Design review of the part built by this model. Coordinates are the model's own, in mm. Face numbers are marked on the shaded views. A direction names the side the tool comes from. Coordinates: 2 decimals unless noted, no trailing zeros. Order: outer loops, then holes, each group sorted by start corner. A loop starts at its lowest first (then second) coordinate and runs counter-clockwise, first axis right, second up. Notation, with made-up numbers: (23, 74.5) -> (68, 74.5) arc R17 ccw to (68, 83.5) -> close; hole circle Ø8 at (48.25, 78.25). An arc over 180 degrees is marked (long way). Use a Markdown table: item, result. Add a question column.
Q1. Machinability: for the marked faces 4 and 5, which of the approach directions +Z, -Z, +X, -X, +Y, -Y give a long, thin tool a straight path to every point of the face, cutting with its end or side? Answer none if there is none.
Q2. The part is to be moulded in two halves that separate along Y. For the marked faces 1, 2 and 3, say which applies: pulls with the +Y half, pulls with the -Y half, needs draft (parallel to the pull), parting line crosses it, or undercut.
Q3. Add section C-C (y = 2). State the section outline as (x, z) points, then the cut area to 3 significant figures.
Q4. Add section A-A (x = 0). State the section outline as (y, z) points.
Q5. Insertion check: pin 1 (1 mm diameter, centred on x = 2, z = -2.5, fed in from +Y); pin 2 (9 mm diameter, centred on x = 0, y = 0, fed in from +Z); pin 3 (1.5 mm diameter, centred on y = 6, z = -1.5, fed in from -X). Each pin has a flat end and moves straight along its axis. Give the tip position at first contact, or say it passes through.
Q6. Wall thickness on probe 1 along Y at (x, z) = (0, -0.55); probe 2 along Y at (x, z) = (0, -1.8); probe 3 along Y at (x, z) = (-0.25, -0.15): over which ranges is each line inside the solid? List them lowest first.
Q7. Add section B-B (z = -2.7). State the section outline as (x, y) points, then the cut area to 3 significant figures.
Q8. Add section D-D (x = 3.25). State the section outline as (y, z) points, then the cut area to 3 significant figures.
from build123d import *

# Parameters (mm, degrees)
F0_R         = 2.75
F1_DEPTH     = 3
F2_DEPTH     = 1.5
F3_T4_DEPTH  = 26.4678686971
F3_S5_R      = 9
F3_T6_DEPTH  = 15
F3_T10_DEPTH = 20.3478228694
F3_S11_R     = 9
F3_T12_DEPTH = 12
F3_T16_DEPTH = 26.4678686971
F3_S17_R     = 9
F3_T18_DEPTH = 15
F3_T22_DEPTH = 20.3478228694
F3_S23_R     = 9
F3_T24_DEPTH = 12


# Not quite as in the source:
# - a fillet or chamfer that OpenCascade refuses, or shapes differently, is made with other operations: its cross-section is extruded or revolved along the edge and cut away or added


with BuildPart() as f1:
    # F0 (on Top) → F1 (new body)
    with BuildSketch(Plane.XY):
        with BuildLine():
            Line((-5.3326822519, 7.25), (5.3326822519, 7.25))
            ThreePointArc((5.3326822519, 7.25), (0, 9), (-5.3326822519, 7.25))
        make_face()
        with BuildLine():
            Line((-8.3927051658, 3.25), (8.3927051658, 3.25))
            ThreePointArc((8.3927051658, 3.25), (7.1481861295, 5.4684033372), (5.3326822519, 7.25))
            Line((5.3326822519, 7.25), (-5.3326822519, 7.25))
            ThreePointArc((-5.3326822519, 7.25), (-7.1481861295, 5.4684033372), (-8.3927051658, 3.25))
        make_face()
        with BuildLine():
            ThreePointArc((5.3326822519, -7.25), (7.1481861295, -5.4684033372), (8.3927051658, -3.25))
            Line((8.3927051658, -3.25), (-8.3927051658, -3.25))
            ThreePointArc((-8.3927051658, -3.25), (-7.1481861295, -5.4684033372), (-5.3326822519, -7.25))
            Line((-5.3326822519, -7.25), (5.3326822519, -7.25))
        make_face()
        with BuildLine():
            ThreePointArc((-5.3326822519, -7.25), (0, -9), (5.3326822519, -7.25))
            Line((5.3326822519, -7.25), (-5.3326822519, -7.25))
        make_face()
        with BuildLine():
            ThreePointArc((8.3927051658, -3.25), (8.8468736425, -1.6531263575), (9, 0))
            ThreePointArc((9, 0), (8.8468736425, 1.6531263575), (8.3927051658, 3.25))
            Line((8.3927051658, 3.25), (-8.3927051658, 3.25))
            ThreePointArc((-8.3927051658, 3.25), (-9, 0), (-8.3927051658, -3.25))
            Line((-8.3927051658, -3.25), (8.3927051658, -3.25))
        make_face()
        Circle(F0_R, mode=Mode.SUBTRACT)
    extrude(amount=-F1_DEPTH)

    # F0 (on Top) → F2 (cut)
    with BuildSketch(Plane.XY):
        with BuildLine():
            Line((-8.3927051658, 3.25), (8.3927051658, 3.25))
            ThreePointArc((8.3927051658, 3.25), (7.1481861295, 5.4684033372), (5.3326822519, 7.25))
            Line((5.3326822519, 7.25), (-5.3326822519, 7.25))
            ThreePointArc((-5.3326822519, 7.25), (-7.1481861295, 5.4684033372), (-8.3927051658, 3.25))
        make_face()
        with BuildLine():
            ThreePointArc((5.3326822519, -7.25), (7.1481861295, -5.4684033372), (8.3927051658, -3.25))
            Line((8.3927051658, -3.25), (-8.3927051658, -3.25))
            ThreePointArc((-8.3927051658, -3.25), (-7.1481861295, -5.4684033372), (-5.3326822519, -7.25))
            Line((-5.3326822519, -7.25), (5.3326822519, -7.25))
        make_face()
    extrude(amount=-F2_DEPTH, mode=Mode.SUBTRACT)

    # F3: fillet of radius 2 on 4 edges, made by hand


with BuildPart() as f3_tool2:
    # F3_s3 → F3_t4 (new body)
    with BuildSketch(Plane.YZ.offset(-13.2339343486)):
        with BuildLine():
            ThreePointArc((3.25, 0), (3.9617468017, -1.0811388301), (5.1864916731, -1.5))
            Line((5.1864916731, -1.5), (3.25, -1.5))
            Line((3.25, -1.5), (3.25, 0))
        make_face()
    extrude(amount=F3_T4_DEPTH)

    # F3_s5 → F3_t6 (intersect, symmetric)
    with BuildSketch(Plane.XY.offset(-0.8)):
        Circle(F3_S5_R)
    extrude(amount=F3_T6_DEPTH, both=True, mode=Mode.INTERSECT)


with BuildPart() as f1_1:
    add(f1.part)

    # F3_t1: union F3_tool2
    add(f3_tool2.part)


with BuildPart() as f3_tool8:
    # F3_s9 → F3_t10 (new body)
    with BuildSketch(Plane.YZ.offset(10.1739114347)):
        with BuildLine():
            ThreePointArc((5.3135083269, -1.5), (6.5382531983, -1.0811388301), (7.25, 0))
            Line((7.25, 0), (7.25, -1.5))
            Line((7.25, -1.5), (5.3135083269, -1.5))
        make_face()
    extrude(amount=-F3_T10_DEPTH)

    # F3_s11 → F3_t12 (intersect, symmetric)
    with BuildSketch(Plane.XY.offset(-0.8)):
        Circle(F3_S11_R)
    extrude(amount=F3_T12_DEPTH, both=True, mode=Mode.INTERSECT)


with BuildPart() as f1_2:
    add(f1_1.part)

    # F3_t7: union F3_tool8
    add(f3_tool8.part)


with BuildPart() as f3_tool14:
    # F3_s15 → F3_t16 (new body)
    with BuildSketch(Plane.YZ.offset(13.2339343486)):
        with BuildLine():
            ThreePointArc((-3.25, 0), (-3.9617468017, -1.0811388301), (-5.1864916731, -1.5))
            Line((-5.1864916731, -1.5), (-3.25, -1.5))
            Line((-3.25, -1.5), (-3.25, 0))
        make_face()
    extrude(amount=-F3_T16_DEPTH)

    # F3_s17 → F3_t18 (intersect, symmetric)
    with BuildSketch(Plane.XY.offset(-0.8)):
        Circle(F3_S17_R)
    extrude(amount=F3_T18_DEPTH, both=True, mode=Mode.INTERSECT)


with BuildPart() as f1_3:
    add(f1_2.part)

    # F3_t13: union F3_tool14
    add(f3_tool14.part)


with BuildPart() as f3_tool20:
    # F3_s21 → F3_t22 (new body)
    with BuildSketch(Plane.YZ.offset(-10.1739114347)):
        with BuildLine():
            ThreePointArc((-5.3135083269, -1.5), (-6.5382531983, -1.0811388301), (-7.25, 0))
            Line((-7.25, 0), (-7.25, -1.5))
            Line((-7.25, -1.5), (-5.3135083269, -1.5))
        make_face()
    extrude(amount=F3_T22_DEPTH)

    # F3_s23 → F3_t24 (intersect, symmetric)
    with BuildSketch(Plane.XY.offset(-0.8)):
        Circle(F3_S23_R)
    extrude(amount=F3_T24_DEPTH, both=True, mode=Mode.INTERSECT)


with BuildPart() as f1_4:
    add(f1_3.part)

    # F3_t19: union F3_tool20
    add(f3_tool20.part)


solid = f1_4.part
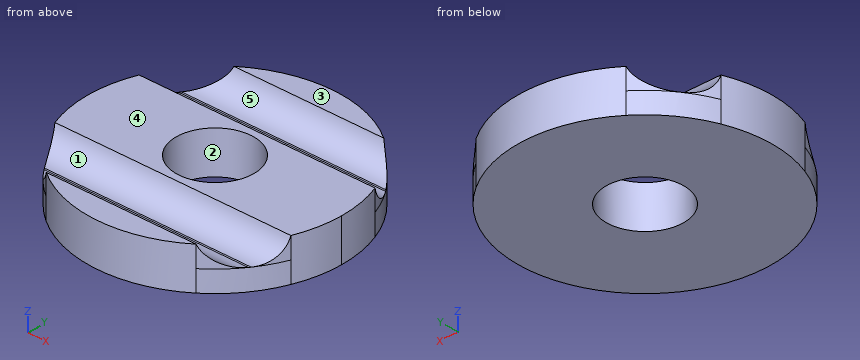
Established:
| question | item | result |
|---|---|---|
| 1 | face 4 | +Z, +X, -X, +Y, -Y |
| 1 | face 5 | +Z, +X, -X |
| 2 | face 1 | undercut |
| 2 | face 2 | undercut |
| 2 | face 3 | needs draft |
| 3 | outline | (-8.77, -3) -> (-1.89, -3) -> (-1.89, 0) -> (-8.77, 0) -> close; (1.89, -3) -> (8.77, -3) -> (8.77, 0) -> (1.89, 0) -> close |
| 3 | area | 41.3 mm^2 |
| 4 | outline | (-9, -3) -> (-2.75, -3) -> (-2.75, 0) -> (-3.25, 0) arc R2 cw to (-5.19, -1.5) -> (-5.31, -1.5) arc R2 cw to (-7.25, 0) -> (-9, 0) -> close; (2.75, -3) -> (9, -3) -> (9, 0) -> (7.25, 0) arc R2 cw to (5.31, -1.5) -> (5.19, -1.5) arc R2 cw to (3.25, 0) -> (2.75, 0) -> close |
| 5 | pin 1 | y = 8.87 |
| 5 | pin 2 | z = 0 |
| 5 | pin 3 | x = -7.31 |
| 6 | probe 1 | -9 to -7.02, -3.48 to -2.75, 2.75 to 3.48, 7.02 to 9 |
| 6 | probe 2 | -9 to -2.75, 2.75 to 9 |
| 6 | probe 3 | -9 to -7.2, -3.3 to -2.74, 2.74 to 3.3, 7.2 to 9 |
| 7 | outline | circle Ø18 at (0, 0); hole circle Ø5.5 at (0, 0) |
| 7 | area | 231 mm^2 |
| 8 | outline | (-8.39, -3) -> (8.39, -3) -> (8.39, 0) -> (7.25, 0) arc R2 cw to (5.31, -1.5) -> (5.19, -1.5) arc R2 cw to (3.25, 0) -> (-3.25, 0) arc R2 cw to (-5.19, -1.5) -> (-5.31, -1.5) arc R2 cw to (-7.25, 0) -> (-8.39, 0) -> close |
| 8 | area | 41.4 mm^2 |
